For this review, use the dimensioned drawing (mm, ordinates from the lowest corner) and the shaded views. A direction names the side the tool comes from. Round coordinates to 2 decimals unless told otherwise and drop trailing zeros. Order: outer loops, then holes, each group sorted by start corner. A loop starts at its lowest first (then second) coordinate and runs counter-clockwise, first axis right, second up. Notation, with made-up numbers: (67.5, 73.5) - (98.5, 73.5) arc R30 ccw to (98.5, 108.5) - close; hole circle Ø2 at (35, 87.25). An arc over 180 degrees is marked (long way). Write each question's results on one line, items separated by ' | '. Start each with the question number.
(1) For L1, parallel to Z at x = 5.08, y = 6.75 (1 decimal); L2, parallel to Z at x = 5, y = 4.75; L3, parallel to Y at x = 4.5, z = 13.5, list the stretches that pass through material, from the lowest coordinate up. Write a range as from..to.
(2) Insertion check: pin 1 Ø5 at (y, z) = (5, 39.5) entering from +X; pin 2 Ø8 at (x, z) = (20.5, 42.5) entering from +Y; pin 3 Ø4 at (y, z) = (4.5, 57) entering from -X; pin 4 Ø2 at (x, y) = (24.5, 6) entering from -Z. Each pin has a flat end and moves straight along its axis. Give the tip position at first contact, or say it passes through.
(3) Take a section at B-B, the plane x = 5.08. Give the number of separate pieces and of enclosed holes in the cut face, plus the area to 3 significant figures.
(4) Take a section at A-A, the plane y = 9.5. Give the boundary of the cut face in (x, z) (1 decimal).
(5) Take a section at D-D, the plane y = 3.5. Give the boundary of the cut face in (x, z) (1 decimal).
(6) Take a section at C-C, the plane z = 32. Give the boundary of the cut face in (x, y).
(7) For the marked faces 1, 2 and 3, list the 3-axis set-ups (+Z, -Z, +X, -X, +Y, -Y) from which the entire face can be reached by the end or side of a thin tool; tool diameter is ignored.
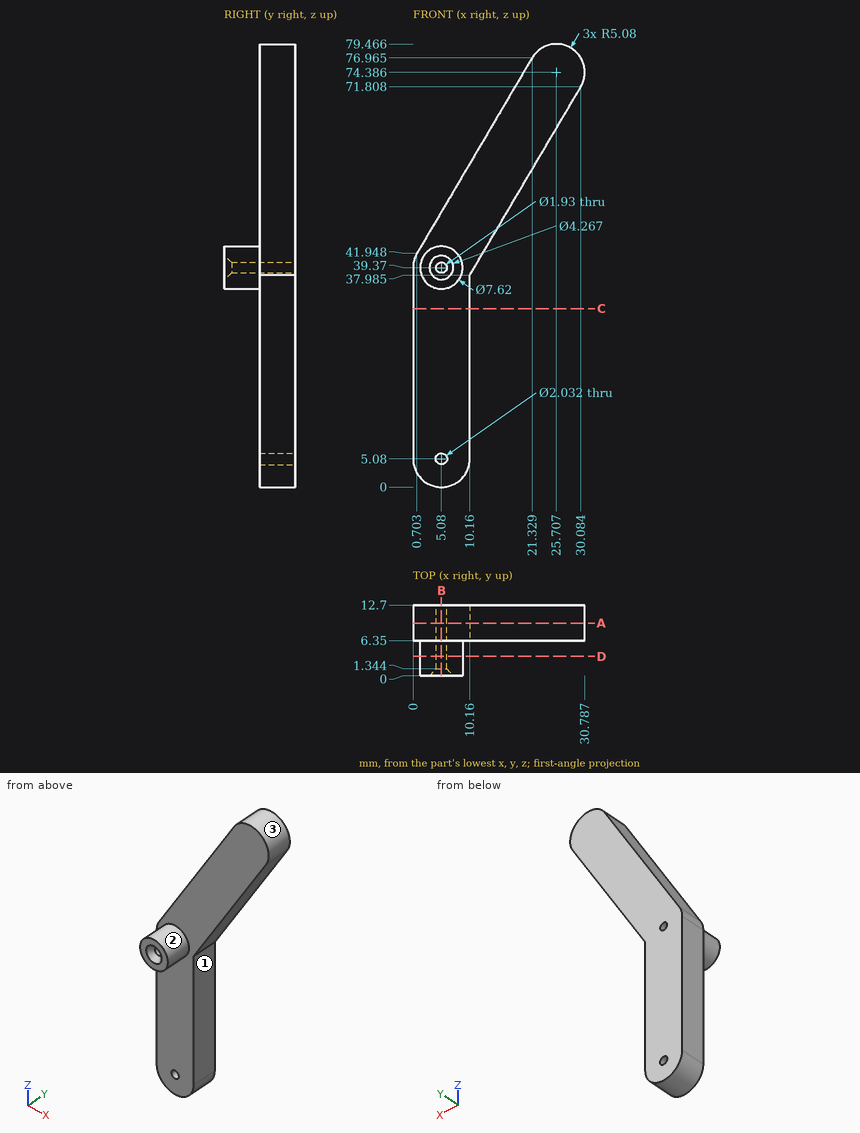
Results below:
1) L1: z = 0..4.1, 6.1..38.4, 40.3..49.4 | L2: z = 35.56..38.41, 40.33..43.18 | L3: y = 6.35..12.7
2) pin 1: stops at x = 12.29 | pin 2: passes through | pin 3: stops at x = 9.12 | pin 4: stops at z = 60.74
3) separate pieces: 3 | enclosed holes: 0 | area: 323 mm^2
4) outline: (0, 5.1) arc R5.1 ccw to (10.2, 5.1) - (10.2, 38) - (30.1, 71.8) arc R5.1 ccw to (21.3, 77) - (0.7, 41.9) arc R5.1 ccw to (0, 39.4) - close; hole circle Ø2 at (5.1, 5.1); hole circle Ø1.9 at (5.1, 39.4)
5) outline: circle Ø7.6 at (5.1, 39.4); hole circle Ø1.9 at (5.1, 39.4)
6) outline: (0, 6.35) - (10.16, 6.35) - (10.16, 12.7) - (0, 12.7) - close
7) face 1: -Z, +X, +Y, -Y | face 2: -Y | face 3: +Y, -Y
